Part model, mm, in its own coordinate system. Face numbers are marked on the shaded views. A direction names the side the tool comes from. Give positions to 0.01 mm unless a question says otherwise; leave off trailing zeros. Write each loop counter-clockwise with the first axis right and the second up, starting at its lowest first coordinate (ties: lowest second). Pieces come first, ordered by that corner, then holes. Notation, with made-up numbers: M -21.5,76 L -1.5,76 A11 cw -1.5,94 Z; hole C 59,56.5 d3. An arc over 180 degrees is marked long. Answer as CSV lines item,"result". Start each with the question number.
1) Slice it at B-B, the plane z = 0. Give the cut face in (x, y), plus the area to 4 significant figures.
2) Mould opens along Z. For the marked faces 1 and 2 say: pulls with the +Z half, pulls with the -Z half, needs draft (parallel to the pull), parting line crosses it, or undercut.
3) Slice it at C-C, the plane x = 60. Give the cut face in (y, z), plus the area to 3 significant figures.
4) Pin check, flat tip, straight feed: pin 1 Ø4.5 at (x, z) = (60, 0) entering from +Y. Stop position of the tip, or through.
5) Tool access for the marked faces 3 and 4: list every direction of +Z, -Z, +X, -X, +Y, -Y with a clear straight run to the whole face (end or side of a thin tool).
6) Wall check: line 1 along X through (y, z) = (5.8, 0); line 2 along X through (y, z) = (2.3, 0); line 3 along Z through (x, y) = (0, 2). Give the ranges that are in metal, low to high. Write a range as from..to.
7) Slice it at D-D, the plane x = 29. Give the cut face in (y, z), plus the area to 3 significant figures.
8) Slice it at A-A, the plane y = 1.5. Give the cut face in (x, z), plus the area to 3 significant figures.
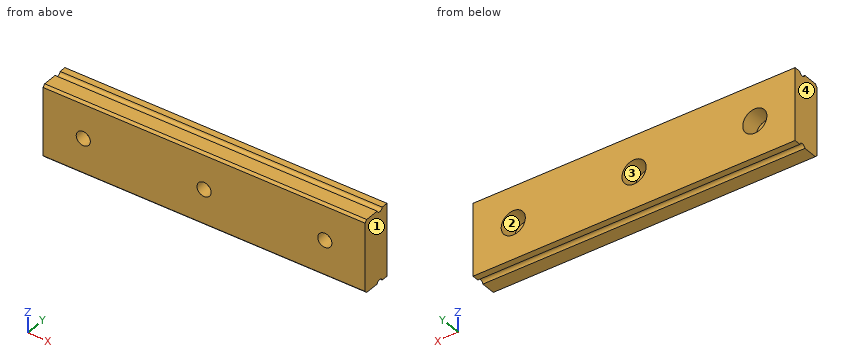
Autodesk Inventor part; units mm, degrees
ref_plane "rail_XY" through (-10, 0, 0) normal (1, 0, 0) x (0, 0, -1)
ref_plane "rail_YZ" through (-10, 0, 0) normal (0, 0, -1) x (0, 1, 0)
ref_plane "rail_ZX" through (-10, 0, 0) normal (0, 1, 0) x (1, 0, 0)
sketch "Sketch_1" plane through (-10, 0, 0) normal (1, 0, 0) x (0, 0, -1)
  arc A0 (-9, 4.1354) -> (-9, 5.8646) centre (-9.25, 5) ccw
  line L0 (-9, 4.1354) -> (-9, 0.57)
  line L1 (-9, 0.57) -> (-8.43, 0)
  line L2 (-8.43, 0) -> (8.43, 0)
  line L3 (8.43, 0) -> (9, 0.57)
  line L4 (9, 0.57) -> (9, 4.1354)
  arc A1 (9, 5.8646) -> (9, 4.1354) centre (9.25, 5) ccw
  line L5 (9, 5.8646) -> (9, 7.5)
  line L6 (9, 7.5) -> (-9, 7.5)
  line L7 (-9, 7.5) -> (-9, 5.8646)
extrude "Extrusion1" add sketch "Sketch_1" along normal blind 80
sketch "Sketch2" plane through (-10, 7.5, 9) normal (0, 1, 0) x (1, 0, 0)
  point P0 (10, 9)
hole "Hole1" at (0, 7.5, 0) direction (0, -1, 0) diameter 3.5 depth 7.5 counterbore diameter 6 counterbore depth 4.5
pattern_linear "Rectangular Pattern1" count 3 spacing 30 along (1, 0, 0) of "Hole1"
ref_plane "rail_XY" through (-10, 0, 0) normal (1, 0, 0) x (0, 0, -1)
ref_plane "rail_YZ" through (-10, 0, 0) normal (0, 0, -1) x (0, 1, 0)
ref_plane "rail_ZX" through (-10, 0, 0) normal (0, 1, 0) x (1, 0, 0)
properties part number "SEBS 9WA UU1T1-80P"
Found:
1,outline,"M -10,0 L -1.75,0 L -1.75,3 L -3,3 L -3,7.5 L -10,7.5 Z; M 1.75,0 L 28.25,0 L 28.25,3 L 27,3 L 27,7.5 L 3,7.5 L 3,3 L 1.75,3 Z; M 31.75,0 L 58.25,0 L 58.25,3 L 57,3 L 57,7.5 L 33,7.5 L 33,3 L 31.75,3 Z; M 61.75,0 L 70,0 L 70,7.5 L 63,7.5 L 63,3 L 61.75,3 Z"
1,area,"487.5 mm²"
2,face 1,"needs draft"
2,face 2,"undercut"
3,outline,"M 0,-8.43 L 0.57,-9 L 4.14,-9 A0.9 cw 5.86,-9 L 7.5,-9 L 7.5,-3 L 3,-3 L 3,-1.75 L 0,-1.75 Z; M 0,1.75 L 3,1.75 L 3,3 L 7.5,3 L 7.5,9 L 5.86,9 A0.9 cw 4.14,9 L 0.57,9 L 0,8.43 Z"
3,area,"95.5 mm²"
4,pin 1,"y = 3"
5,face 3,"+Y"
5,face 4,"+Z, -Z, -X, +Y, -Y"
6,line 1,"-10..-3, 3..27, 33..57, 63..70"
6,line 2,"-10..-1.75, 1.75..28.25, 31.75..58.25, 61.75..70"
6,line 3,"-9..-1.75, 1.75..9"
7,outline,"M 0,-8.43 L 0.57,-9 L 4.14,-9 A0.9 cw 5.86,-9 L 7.5,-9 L 7.5,-2.83 L 3,-2.83 L 3,-1.44 L 0,-1.44 Z; M 0,1.44 L 3,1.44 L 3,2.83 L 7.5,2.83 L 7.5,9 L 5.86,9 A0.9 cw 4.14,9 L 0.57,9 L 0,8.43 Z"
7,area,"98.9 mm²"
8,outline,"M -10,-9 L 70,-9 L 70,9 L -10,9 Z; hole C 0,0 d3.5; hole C 30,0 d3.5; hole C 60,0 d3.5"
8,area,"1,410 mm²"
